Here's how the part is built. I have some questions about the finished solid (model axes, mm). A direction names the side the tool comes from. Give positions to 0.01 mm unless a question says otherwise; leave off trailing zeros. Loops run counter-clockwise (first coordinate to the right, second up) from the corner with the lowest first, then second, coordinate; pieces in that order, holes last. Notation, with made-up numbers: (48, 17.5) - (101, 17.5) arc R20 ccw to (101, 32.5) - close; hole circle Ø9 at (78.25, -33.5). An arc over 180 degrees is marked (long way). Use one line per item in the form item = value.
from build123d import *

# Parameters (mm, degrees)
F0_W     = 73.3068473637
F0_H     = 45.9237424657
F1_DEPTH = 254
F2_R     = 86.0682803243
F3_DEPTH = 25.4
F4_R     = 27.0619318238
F4_R_2   = 24.0411397983
F5_DEPTH = 12.7


with BuildPart() as f1:
    # F0 (on Front) → F1 (new body)
    with BuildSketch(Plane.XZ):
        with Locations((-1.5688221902, 14.5472721197)):
            Rectangle(F0_W, F0_H)
    extrude(amount=F1_DEPTH)

    # F2 (on face) → F3 (join)
    with BuildSketch(Plane.XY.offset(37.5091433525)):
        with Locations((0, -131.3995718956)):
            Circle(F2_R)
    extrude(amount=F3_DEPTH)

    # F4 (on face) → F5 (join)
    with BuildSketch(Plane(origin=(-38.222245872, 0, 0), x_dir=(0, -1, 0), z_dir=(-1, 0, 0))):
        with Locations((234.2655062675, 12.6427337527)):
            Circle(F4_R)
        with Locations((35.7813984156, 12.6427337527)):
            Circle(F4_R_2)
    extrude(amount=F5_DEPTH)


solid = f1.part
(1) If we section it at D-D (z = 18): List the corners of the cut face in (x, y) for me, plus the area to 3 significant figures.
Geometry says:
outline = (-50.92, -260.79) - (-38.22, -260.79) - (-38.22, -254) - (35.08, -254) - (35.08, 0) - (-38.22, 0) - (-38.22, -12.34) - (-50.92, -12.34) - (-50.92, -59.22) - (-38.22, -59.22) - (-38.22, -207.74) - (-50.92, -207.74) - close
area = 19,900 mm²
(2) If I drill on probe 1 along Z at (x, y) = (2.5, -15); probe 2 along Z at (x, y) = (-6, -68); probe 3 along X at (y, z) = (-171, -8), over which ranges is the centre line in solid material (lowest first)?
Geometry says:
probe_1 = -8.41 to 37.51
probe_2 = -8.41 to 62.91
probe_3 = -38.22 to 35.08
(3) For P1, Ø10, axis at y = -209.5, z = 30, coming from the -X side; P2, Ø5, axis at y = -161.5, z = 21, coming from the -X side; P3, Ø12, axis at y = -85, z = 49.5, coming from the -X side, each with a flat end and sliding along its axis, tell me the tip position at first contact or that it passes through.
Geometry says:
P1 = -50.92
P2 = -38.22
P3 = -76
(4) If we section it at A-A (x = 0): List the corners of the cut face in (y, z) for me.
Geometry says:
outline = (-254, -8.41) - (0, -8.41) - (0, 37.51) - (-45.33, 37.51) - (-45.33, 62.91) - (-217.47, 62.91) - (-217.47, 37.51) - (-254, 37.51) - close
(5) If we section it at B-B (z = 6.5): List the corners of the cut face in (x, y) for me, plus the area to 3 significant figures.
Geometry says:
outline = (-50.92, -260.62) - (-38.22, -260.62) - (-38.22, -254) - (35.08, -254) - (35.08, 0) - (-38.22, 0) - (-38.22, -12.54) - (-50.92, -12.54) - (-50.92, -59.02) - (-38.22, -59.02) - (-38.22, -207.91) - (-50.92, -207.91) - close
area = 19,900 mm²
(6) If we section it at C-C (y = -164.5): List the corners of the cut face in (x, z) for me, plus the area to 3 significant figures.
Geometry says:
outline = (-79.45, 37.51) - (-38.22, 37.51) - (-38.22, -8.41) - (35.08, -8.41) - (35.08, 37.51) - (79.45, 37.51) - (79.45, 62.91) - (-79.45, 62.91) - close
area = 7,400 mm²
(7) For faces 1 (the flat face through (-38.222, -251, 36)), 2 (the flat face through (55, -130, 37.509)), 3 (the flat face through (-38.222, -257, 13)), 4 (the cylindrical face through (-18.66, -215.42, 50.03)), 5 (the cylindrical face through (-44.48, -207.23, 13.83)), which set-ups out of +Z, -Z, +X, -X, +Y, -Y let a thin tool reach every point of the face, with its end or its side?
Geometry says:
face_1 = +Z, -X, -Y
face_2 = -Z, +X, +Y, -Y
face_3 = +Z, -Z, +X, -Y
face_4 = +Z
face_5 = -X
(8) Thinking about a two-plate mould opening in Y: for faces 6 (the flat face through (35.085, -125, 14)), 7 (the flat face through (-2, 0, 15)), 8 (the cylindrical face through (-44.483, -16.703, -1.986)), 9 (the flat face through (-2, -254, 15)), which applies, pulls with the +Y half, pulls with the -Y half, needs draft (parallel to the pull), parting line crosses it, or undercut?
Geometry says:
face_6 = needs draft
face_7 = pulls with the +Y half
face_8 = undercut
face_9 = pulls with the -Y half
